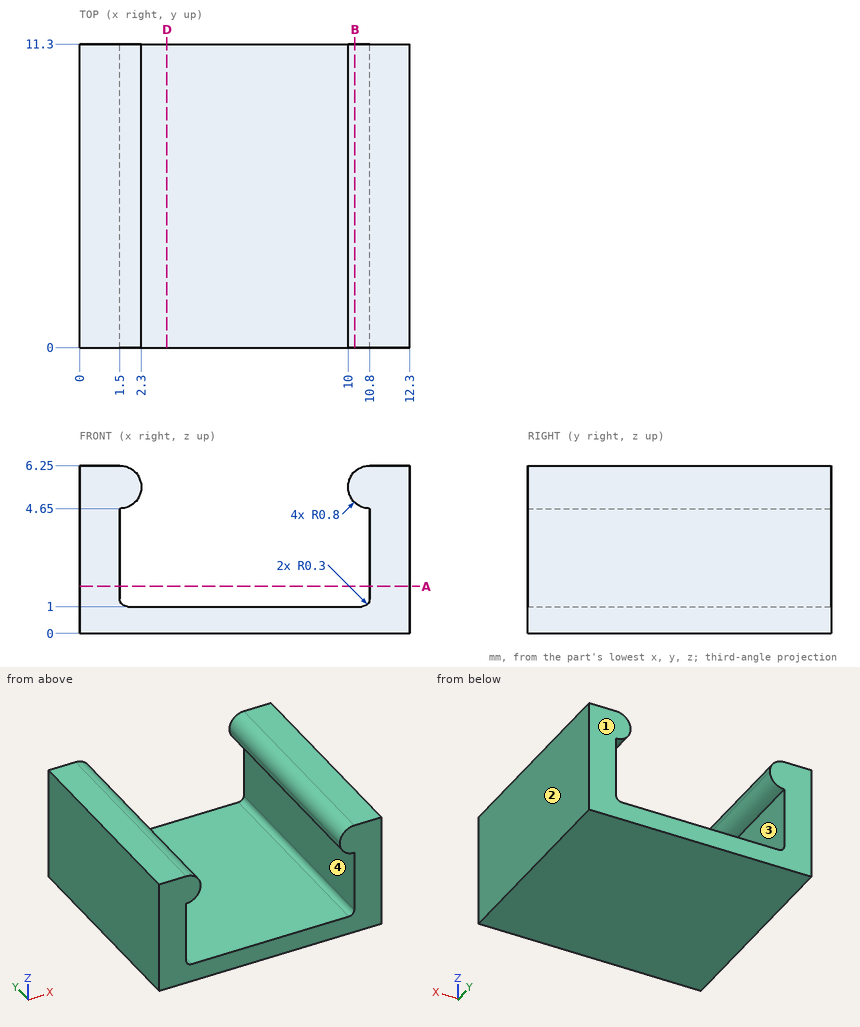
Here's the drawing with two shaded views (mm, measured from the low corner). I have some questions. Coordinates: 2 decimals unless noted, no trailing zeros. Order: outer loops, then holes, each group sorted by start corner. A loop starts at its lowest first (then second) coordinate and runs counter-clockwise, first axis right, second up.
Item 1: If we section it at A-A, the plane z = 1.75: List the corners of the cut face in (x, y) for me.
Response values:
outline: (0, 0) - (1.5, 0) - (1.5, 11.3) - (0, 11.3) - close; (10.8, 0) - (12.3, 0) - (12.3, 11.3) - (10.8, 11.3) - close
Item 2: I need wall thicknesses on probe 1 along X at (y, z) = (5.5, 4); probe 2 along Z at (x, y) = (3.75, 6.25); probe 3 along X at (y, z) = (3.5, 5.5). Which ranges of each line are inside material? Lowest first, please.
Response values:
probe 1: x = 0 to 1.5, 10.8 to 12.3
probe 2: z = 0 to 1
probe 3: x = 0 to 2.3, 10 to 12.3
Item 3: If we section it at B-B, the plane x = 10.25: List the corners of the cut face in (y, z) for me.
Response values:
outline: (0, 0) - (11.3, 0) - (11.3, 1) - (0, 1) - close; (0, 4.87) - (11.3, 4.87) - (11.3, 6.03) - (0, 6.03) - close
Item 4: If we section it at D-D, the plane x = 3.25: List the corners of the cut face in (y, z) for me, then the cut area to 3 significant figures.
Response values:
outline: (0, 0) - (11.3, 0) - (11.3, 1) - (0, 1) - close
area: 11.3 mm2
Item 5: Thinking about a two-plate mould opening in X: for the marked faces 1, 2, 3 and 4, which applies, pulls with the +X half, pulls with the -X half, needs draft (parallel to the pull), parting line crosses it, or undercut?
Response values:
face 1: needs draft
face 2: pulls with the +X half
face 3: undercut
face 4: undercut
